from build123d import *

# Parameters (mm, degrees)
F1_DEPTH    = 88.9
F2_T        = -2.54
F3_T1_DEPTH = 103.5646968374
F3_T3_DEPTH = 79.9330955154
F4_T1_DEPTH = 103.5646968374
F4_T3_DEPTH = 79.9330955154
F5_T1_DEPTH = 103.5646968374
F5_T3_DEPTH = 79.9330955154
F6_DEPTH    = 22.86


# Not quite as in the source:
# - a fillet or chamfer that OpenCascade refuses, or shapes differently, is made with other operations: its cross-section is extruded or revolved along the edge and cut away or added


with BuildPart() as f1:
    # F0 (on Right) → F1 (new body)
    with BuildSketch(Plane.YZ):
        Polygon((-15.657663601, 52.2369225457), (-53.0673337406, 12.5585268304), (-37.4096701396, -39.6783957152), (15.657663601, -52.2369225457), (53.0673337406, -12.5585268304), (37.4096701396, 39.6783957152), align=None)
    extrude(amount=F1_DEPTH)

    # F2
    f2_openings = [f1.faces().sort_by_distance(p)[0] for p in [
        (0, 0, 0),
    ]]
    offset(amount=F2_T, openings=f2_openings)

    # F3: fillet of radius 5.08 on 4 edges, made by hand

    # F3_s2 → F3_t1 (cut)
    with BuildSketch(Plane.YZ.offset(-7.3323484187)):
        with BuildLine():
            ThreePointArc((-12.8035569199, 51.5614905463), (-15.4320203518, 51.484134056), (-17.6696582116, 50.1029096544))
            Line((-17.6696582116, 50.1029096544), (-15.657663601, 52.2369225457))
            Line((-15.657663601, 52.2369225457), (-12.8035569199, 51.5614905463))
        make_face()
        with BuildLine():
            ThreePointArc((-51.05533913, 14.6925397217), (-52.3025781603, 12.3775453716), (-52.22522167, 9.7490819397))
            Line((-52.22522167, 9.7490819397), (-53.0673337406, 12.5585268304))
            Line((-53.0673337406, 12.5585268304), (-51.05533913, 14.6925397217))
        make_face()
    extrude(amount=F3_T1_DEPTH, mode=Mode.SUBTRACT)

    # F3_s4 → F3_t3 (cut)
    with BuildSketch(Plane(origin=(0, 27.4170272951, 29.0797447369), x_dir=(1, 0, 0), z_dir=(0, -0.6859993878, -0.7276021165))):
        with BuildLine():
            ThreePointArc((5.08, 47.2270460633), (1.4878975516, 45.7391485117), (0, 42.1470460633))
            Line((0, 42.1470460633), (0, 47.2270460633))
            Line((0, 47.2270460633), (5.08, 47.2270460633))
        make_face()
        with BuildLine():
            ThreePointArc((83.82, 47.2270460633), (87.4121024484, 45.7391485117), (88.9, 42.1470460633))
            Line((88.9, 42.1470460633), (88.9, 47.2270460633))
            Line((88.9, 47.2270460633), (83.82, 47.2270460633))
        make_face()
    extrude(amount=F3_T3_DEPTH, mode=Mode.SUBTRACT)

    # F4: fillet of radius 5.08 on 4 edges, made by hand

    # F4_s2 → F4_t1 (cut)
    with BuildSketch(Plane.YZ.offset(-7.3323484187)):
        with BuildLine():
            ThreePointArc((52.22522167, -9.7490819397), (52.3025781603, -12.3775453716), (51.05533913, -14.6925397217))
            Line((51.05533913, -14.6925397217), (53.0673337406, -12.5585268304))
            Line((53.0673337406, -12.5585268304), (52.22522167, -9.7490819397))
        make_face()
        with BuildLine():
            ThreePointArc((38.2517822101, 36.8689508245), (36.8705578085, 39.1065886844), (34.5555634584, 40.3538277147))
            Line((34.5555634584, 40.3538277147), (37.4096701396, 39.6783957152))
            Line((37.4096701396, 39.6783957152), (38.2517822101, 36.8689508245))
        make_face()
    extrude(amount=F4_T1_DEPTH, mode=Mode.SUBTRACT)

    # F4_s4 → F4_t3 (cut)
    with BuildSketch(Plane(origin=(0, 11.4752840302, -38.2837145023), x_dir=(1, 0, 0), z_dir=(0, -0.2871222228, 0.9578939551))):
        with BuildLine():
            ThreePointArc((5.08, 47.2270460633), (1.4878975516, 45.7391485117), (0, 42.1470460633))
            Line((0, 42.1470460633), (0, 47.2270460633))
            Line((0, 47.2270460633), (5.08, 47.2270460633))
        make_face()
        with BuildLine():
            ThreePointArc((83.82, 47.2270460633), (87.4121024484, 45.7391485117), (88.9, 42.1470460633))
            Line((88.9, 42.1470460633), (88.9, 47.2270460633))
            Line((88.9, 47.2270460633), (83.82, 47.2270460633))
        make_face()
    extrude(amount=F4_T3_DEPTH, mode=Mode.SUBTRACT)

    # F5: fillet of radius 5.08 on 4 edges, made by hand

    # F5_s2 → F5_t1 (cut)
    with BuildSketch(Plane.YZ.offset(-7.3323484187)):
        with BuildLine():
            ThreePointArc((-34.5555634584, -40.3538277147), (-36.8705578085, -39.1065886844), (-38.2517822101, -36.8689508245))
            Line((-38.2517822101, -36.8689508245), (-37.4096701396, -39.6783957152))
            Line((-37.4096701396, -39.6783957152), (-34.5555634584, -40.3538277147))
        make_face()
        with BuildLine():
            ThreePointArc((17.6696582116, -50.1029096544), (15.4320203518, -51.484134056), (12.8035569199, -51.5614905463))
            Line((12.8035569199, -51.5614905463), (15.657663601, -52.2369225457))
            Line((15.657663601, -52.2369225457), (17.6696582116, -50.1029096544))
        make_face()
    extrude(amount=F5_T1_DEPTH, mode=Mode.SUBTRACT)

    # F5_s4 → F5_t3 (cut)
    with BuildSketch(Plane(origin=(0, -38.8923113253, 9.2039697654), x_dir=(1, 0, 0), z_dir=(0, 0.9731216106, -0.2302918386))):
        with BuildLine():
            ThreePointArc((0, 42.1470460633), (1.4878975516, 45.7391485117), (5.08, 47.2270460633))
            Line((5.08, 47.2270460633), (0, 47.2270460633))
            Line((0, 47.2270460633), (0, 42.1470460633))
        make_face()
        with BuildLine():
            ThreePointArc((88.9, 42.1470460633), (87.4121024484, 45.7391485117), (83.82, 47.2270460633))
            Line((83.82, 47.2270460633), (88.9, 47.2270460633))
            Line((88.9, 47.2270460633), (88.9, 42.1470460633))
        make_face()
    extrude(amount=F5_T3_DEPTH, mode=Mode.SUBTRACT)

    # F6 (add): a face of the model
    f6_faces = [f1.faces().sort_by_distance(p)[0] for p in [
        (86.36, 0, 0),
    ]]
    extrude(f6_faces, amount=-F6_DEPTH)


solid = f1.part
Part model, mm, in its own coordinate system. A direction names the side the tool comes from. Give positions to 0.01 mm unless a question says otherwise; leave off trailing zeros. Loops run counter-clockwise (first coordinate to the right, second up) from the corner with the lowest first, then second, coordinate; pieces in that order, holes last. Notation, with made-up numbers: M 3,13 L 51,13 A26 cw 51,32 Z; hole C -25,72 d10. An arc over 180 degrees is marked long. Put each result on its own line as item: value. Start each with the question number.
1) Saw through at D-D (y = 28.5). List the corners of the cut face in (x, z).
2) 3-axis set-ups, long thin cutter, end or side, ignore diameter. For faces 4 (the flat face through (98.573, -32.267, 30.918)), 5 (the flat face through (88.9, -44, -13)), 6 (the flat face through (42.92, 42.91, 12.48)), 7 (the flat face through (43.899, -34.129, 32.646)), 8 (the flat face through (98.57, 42.91, 12.48)): which of +Z, -Z, +X, -X, +Y, -Y reach the whole face in a straight line?
3) Probe probe 1 along X at (y, z) = (-4, -11); probe 2 along Z at (x, y) = (78, 15.5); probe 3 along Y at (x, z) = (40, 18.5). List the from-to ranges inside material, lowest first.
4) Pull direction Y, two halves, no side cores. Call faces 1 (the flat face through (43.828, -45.336, -13.234)), 2 (the flat face through (43.83, 11.21, 45.88)), 3 (the flat face through (42.575, 10.643, 43.403)): +Y half, -Y half, draft (parallel to the pull), parting line (faces both ways), or undercut.
5) Flat gauge pins, fed straight in: pin 1 (3 mm diameter, centred on x = 62.5, z = 37, fed in from +Y); pin 2 (4 mm diameter, centred on x = 40.5, y = 11.5, fed in from +Z); pin 3 (3 mm diameter, centred on x = 20, z = 31.5, fed in from +Y). Where does each tip first touch, or does it go through?
6) Saw through at A-A (x = 68). List the corners of the cut face in (y, z), then the cut area to 3 significant figures.
7) Saw through at B-B (x = 92.5). List the corners of the cut face in (y, z), then the cut area to 3 significant figures.
8) Saw through at C-C (z = -20). List the corners of the cut face in (x, y), then the cut area to 3 significant figures.
Numbers:
1. outline: M 0,-38.62 L 88.9,-38.62 L 88.9,-34.91 L 109.22,-34.91 L 109.22,39.18 L 88.9,39.18 L 88.9,41.79 L 0,41.79 L 0,39.18 L 86.36,39.18 L 86.36,-34.91 L 0,-34.91 Z
2. face 4: +Z, +X, -Y
2. face 5: -Z, +X, -Y
2. face 6: -X
2. face 7: +Z, +X, -X, -Y
2. face 8: +Z, +X, +Y
3. probe 1: 86.36 to 109.22
3. probe 2: -51.46 to -48.7, 42.25 to 44.86
3. probe 3: -47.47 to -43.97, 41.11 to 43.76
4. face 1: -Y half
4. face 2: +Y half
4. face 3: undercut
5. pin 1: y = 38.66
5. pin 2: z = 46.28
5. pin 3: y = 40.31
6. outline: M -52.23,9.75 L -38.25,-36.87 A5.08 ccw -34.56,-40.35 L 12.8,-51.56 A5.08 ccw 17.67,-50.1 L 51.06,-14.69 A5.08 ccw 52.23,-9.75 L 38.25,36.87 A5.08 ccw 34.56,40.35 L -12.8,51.56 A5.08 ccw -17.67,50.1 L -51.06,14.69 A5.08 ccw Z; hole M -50.21,11.88 L -35.4,-37.54 L 14.82,-49.43 L 50.21,-11.88 L 35.4,37.54 L -14.82,49.43 Z
6. area: 800 mm^2
7. outline: M -50.21,11.88 L -35.4,-37.54 L 14.82,-49.43 L 50.21,-11.88 L 35.4,37.54 L -14.82,49.43 Z
7. area: 6,920 mm^2
8. outline: M 0,-43.31 L 88.9,-43.31 L 88.9,-40.66 L 109.22,-40.66 L 109.22,42.56 L 88.9,42.56 L 88.9,46.05 L 0,46.05 L 0,42.56 L 86.36,42.56 L 86.36,-40.66 L 0,-40.66 Z
8. area: 2,450 mm^2
